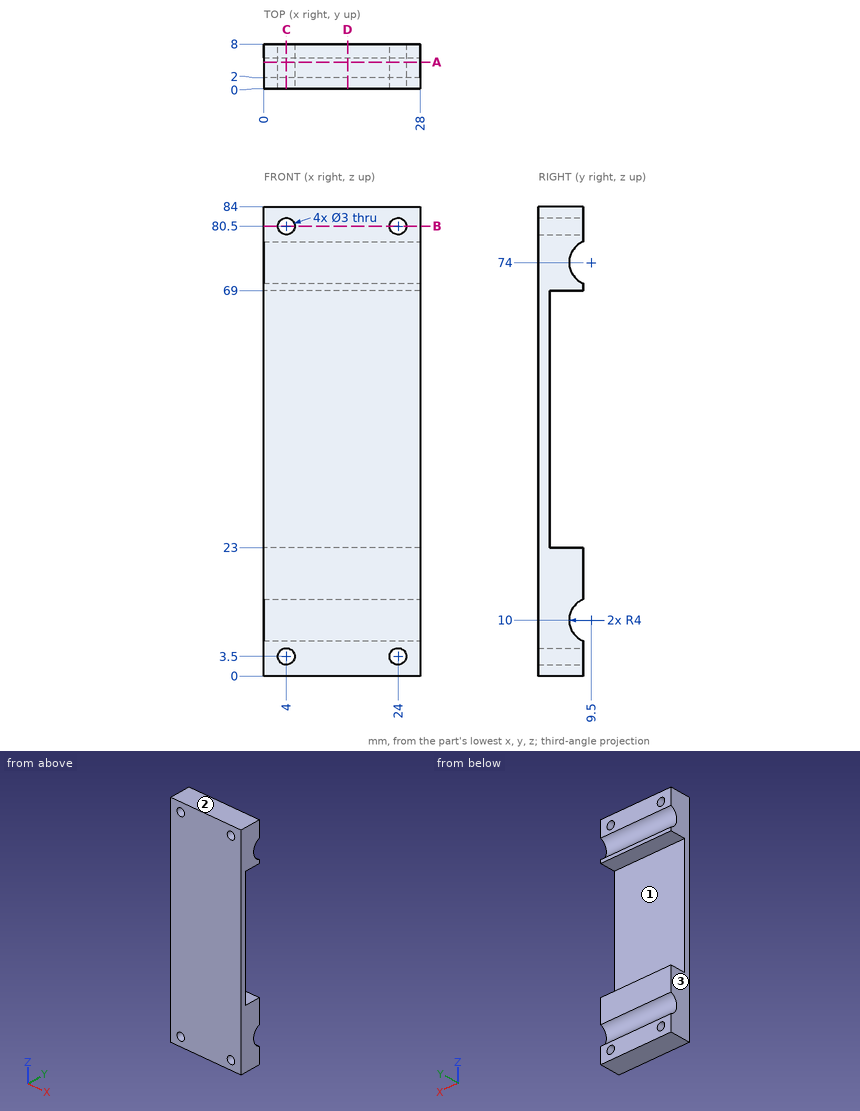
Design review of the part shown in the three views and the two pictorial views. Dimensions are in mm from the part's minimum x, y and z. Round coordinates to 2 decimals unless told otherwise and drop trailing zeros. Write each loop counter-clockwise with the first axis right and the second up, starting at its lowest first coordinate (ties: lowest second). Pieces come first, ordered by that corner, then holes.
Item 1: Clearance check with flat-ended pins moving along their axes: pin 1 Ø8 at (x, z) = (20.5, 33.5) entering from +Y; pin 2 Ø2.5 at (x, z) = (24, 80.5) entering from +Y. State where each tip first meets the part, or that it passes through.
Item 2: We need section A-A on y = 4.75. Write out the cut boundary in (x, z).
Item 3: We need section B-B on z = 80.5. Write out the cut boundary in (x, y).
Item 4: The part is to be moulded in two halves that separate along Z. For the marked faces 1, 2 and 3, say which applies: +Z half, -Z half, draft (parallel to the pull), parting line (faces both ways), or undercut.
Item 5: We need section C-C on x = 4. Write out the cut boundary in (y, z), and give its area (3 significant figures).
Item 6: For probe 1 along Z at (x, y) = (24, 3.25); probe 2 along X at (y, z) = (3.75, 80.5); probe 3 along Z at (x, y) = (24, 0.75), list the stretches that pass through material, from the lowest coordinate up.
Item 7: We need section D-D on x = 15. Write out the cut boundary in (y, z).
Returned:
1. pin 1: stops at y = 2
1. pin 2: passes through
2. outline: (0, 0) - (28, 0) - (28, 23) - (0, 23) - close; (0, 69) - (28, 69) - (28, 84) - (0, 84) - close; hole circle Ø3 at (4, 3.5); hole circle Ø3 at (4, 80.5); hole circle Ø3 at (24, 3.5); hole circle Ø3 at (24, 80.5)
3. outline: (0, 0) - (2.5, 0) - (2.5, 8) - (0, 8) - close; (5.5, 0) - (22.5, 0) - (22.5, 8) - (5.5, 8) - close; (25.5, 0) - (28, 0) - (28, 8) - (25.5, 8) - close
4. face 1: undercut
4. face 2: +Z half
4. face 3: draft
5. outline: (0, 0) - (8, 0) - (8, 2) - (0, 2) - close; (0, 5) - (8, 5) - (8, 6.29) arc R4 cw to (8, 13.71) - (8, 23) - (2, 23) - (2, 69) - (8, 69) - (8, 70.29) arc R4 cw to (8, 77.71) - (8, 79) - (0, 79) - close; (0, 82) - (8, 82) - (8, 84) - (0, 84) - close
5. area: 321 mm2
6. probe 1: z = 0 to 2, 5 to 23, 69 to 79, 82 to 84
6. probe 2: x = 0 to 2.5, 5.5 to 22.5, 25.5 to 28
6. probe 3: z = 0 to 2, 5 to 79, 82 to 84
7. outline: (0, 0) - (8, 0) - (8, 6.29) arc R4 cw to (8, 13.71) - (8, 23) - (2, 23) - (2, 69) - (8, 69) - (8, 70.29) arc R4 cw to (8, 77.71) - (8, 84) - (0, 84) - close
